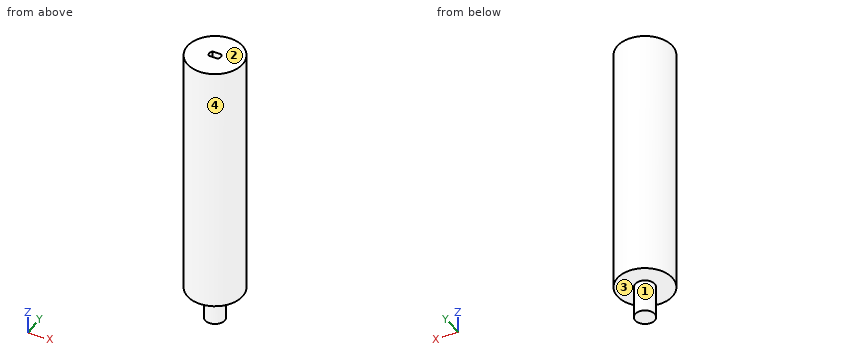
from build123d import *

# Parameters (mm, degrees)
SKETCH2_R           = 12.5
BOSS_EXTRUDE1_DEPTH = 116
SKETCH3_R           = 4.45
BOSS_EXTRUDE2_DEPTH = 15
CUT_EXTRUDE1_DEPTH  = 10


with BuildPart() as part:
    # Sketch2 → Boss-Extrude1 (new body)
    with BuildSketch(Plane.XY):
        Circle(SKETCH2_R)
    extrude(amount=-BOSS_EXTRUDE1_DEPTH)

    # Sketch3 → Boss-Extrude2 (add)
    with BuildSketch(Plane(origin=(0, 0, -116), x_dir=(-1, 0, 0), z_dir=(0, 0, -1))):
        Circle(SKETCH3_R)
    extrude(amount=BOSS_EXTRUDE2_DEPTH)

    # Sketch1 → Cut-Extrude1 (cut)
    with BuildSketch(Plane.XY):
        with BuildLine():
            Line((2.051104302, -1.567413373), (-2.047676004, -1.567413373))
            ThreePointArc((-2.047676004, -1.567413373), (-2.598285851, 0.032586627), (-2.047676004, 1.632586627))
            Line((-2.047676004, 1.632586627), (2.051104302, 1.632586627))
            ThreePointArc((2.051104302, 1.632586627), (2.601714149, 0.032586627), (2.051104302, -1.567413373))
        make_face()
    extrude(amount=-CUT_EXTRUDE1_DEPTH, mode=Mode.SUBTRACT)


solid = part.part
Can you work these out from the model? Positions are in its coordinate system, mm. Face numbers are marked on the shaded views. A direction names the side the tool comes from. Coordinates: 2 decimals unless noted, no trailing zeros. Write each loop counter-clockwise with the first axis right and the second up, starting at its lowest first coordinate (ties: lowest second). Pieces come first, ordered by that corner, then holes.
Q1. Which directions (+Z, -Z, +X, -X, +Y, -Y) give clear straight access to the entire face, cutting with the end or side of a thin tool? Please do the marked faces 3 and 4.
Results found:
face 3: -Z
face 4: +Z, -Z
Q2. For P1, Ø2, axis at x = 1, y = 4.5, coming from the +Z side; P2, Ø5, axis at y = 4, z = -95.5, coming from the -X side; P3, Ø1, axis at x = -1, z = -113, coming from the +Y side; P4, Ø2, axis at x = 3, y = -7.5, coming from the -Z side, each with a flat end and sliding along its axis, tell me the tip position at first contact or that it passes through.
Results found:
P1: stops at z = 0
P2: stops at x = -12.41
P3: stops at y = 12.49
P4: stops at z = -116
Q3. Imagine slicing it at A-A, the plane x = 0. List the corners of the cut face in (y, z) for me, plus the area to 3 significant figures.
Results found:
outline: (-12.5, -116) - (-4.45, -116) - (-4.45, -131) - (4.45, -131) - (4.45, -116) - (12.5, -116) - (12.5, 0) - (1.63, 0) - (1.63, -10) - (-1.57, -10) - (-1.57, 0) - (-12.5, 0) - close
area: 3,000 mm2
Q4. Imagine slicing it at C-C, the plane z = -32. List the corners of the cut face in (x, y) for me, plus the area to 3 significant figures.
Results found:
outline: circle Ø25 at (0, 0)
area: 491 mm2
Q5. Imagine slicing it at B-B, the plane y = 0. List the corners of the cut face in (x, z) for me, plus the area to 3 significant figures.
Results found:
outline: (-12.5, -116) - (-4.45, -116) - (-4.45, -131) - (4.45, -131) - (4.45, -116) - (12.5, -116) - (12.5, 0) - (2.6, 0) - (2.6, -10) - (-2.6, -10) - (-2.6, 0) - (-12.5, 0) - close
area: 2,980 mm2
Q6. Imagine slicing it at D-D, the plane x = -10. List the corners of the cut face in (y, z) for me, plus the area to 3 significant figures.
Results found:
outline: (-7.5, -116) - (7.5, -116) - (7.5, 0) - (-7.5, 0) - close
area: 1,740 mm2
Q7. Please list where these lines run through material, in increasing order: L1, parallel to Z at x = 6.5, y = 1.5; L2, parallel to Y at x = -0.75, z = -47.5; L3, parallel to X at y = -6.5, z = -25.
Results found:
L1: z = -116 to 0
L2: y = -12.48 to 12.48
L3: x = -10.68 to 10.68
Q8. If we mould it in two halves opening along X, with no side actions, what happens to the marked faces 1 and 2? For each: +X half, -X half, draft (parallel to the pull), parting line (faces both ways), or undercut.
Results found:
face 1: parting line
face 2: draft
